Check sheet for the drawn part. Datum: minimum x, y, z corner. Units: mm. Round coordinates to 2 decimals unless told otherwise and drop trailing zeros. Write each loop counter-clockwise with the first axis right and the second up, starting at its lowest first coordinate (ties: lowest second). Pieces come first, ordered by that corner, then holes. Notation, with made-up numbers: (81.25, 68) - (87.25, 68) arc R8 ccw to (87.25, 79) - close; hole circle Ø9 at (37.25, -32). An arc over 180 degrees is marked (long way). Answer as a JSON object with one key per item and string values.
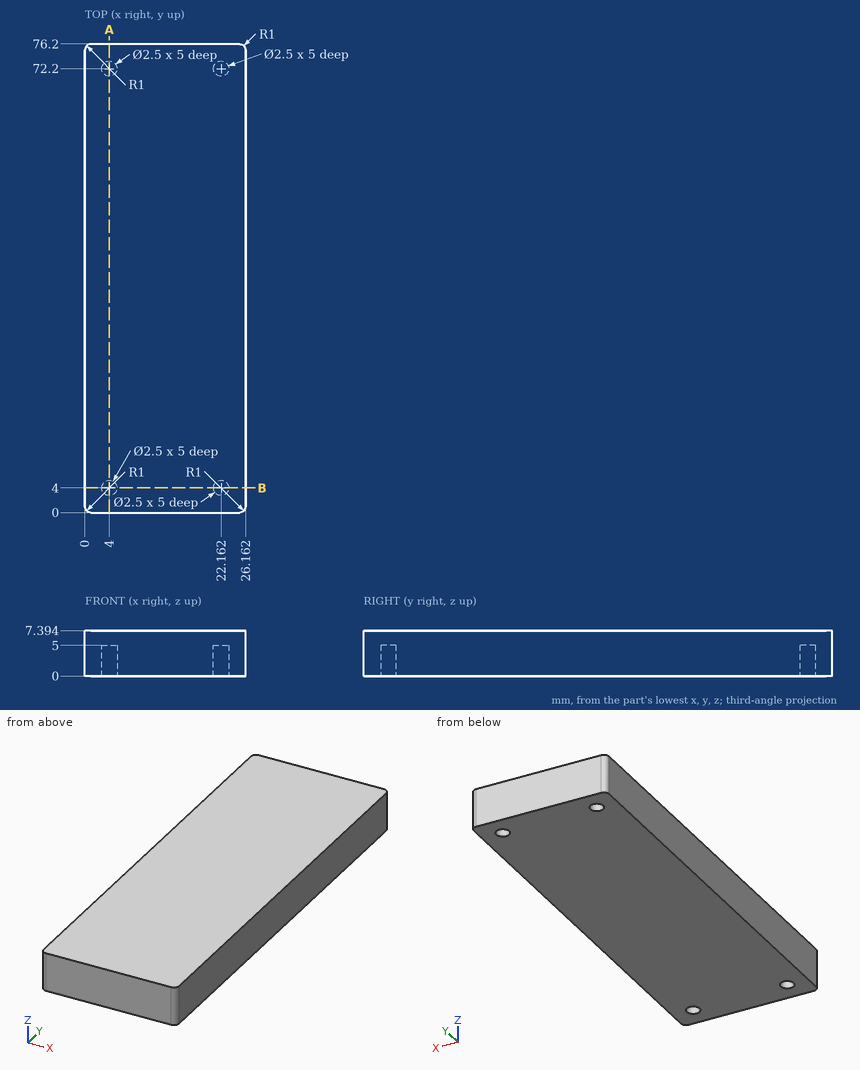
Q1. Section check A-A, the plane x = 4. Record the cut outline in (y, z).
Geometry check:
{"outline": "(0, 0) - (2.75, 0) - (2.75, 5) - (5.25, 5) - (5.25, 0) - (70.95, 0) - (70.95, 5) - (73.45, 5) - (73.45, 0) - (76.2, 0) - (76.2, 7.39) - (0, 7.39) - close"}
Q2. Gauge pin test, flat end, axial feed: P1, Ø2, axis at x = 4, y = 72.2, coming from the -Z side. Record the tip position at first contact, or that the pin passes through.
Geometry check:
{"P1": "stops at z = 5"}
Q3. Material ranges on line 1 along Y through (x, z) = (4, 2.8); line 2 along X through (y, z) = (72.2, 2.35), recorded low to high. Write a range as [from, to].
Geometry check:
{"line 1": "y = [0, 2.75], [5.25, 70.95], [73.45, 76.2]", "line 2": "x = [0, 2.75], [5.25, 20.91], [23.41, 26.16]"}
Q4. Section check B-B, the plane y = 4. Record the cut outline in (x, z).
Geometry check:
{"outline": "(0, 0) - (2.75, 0) - (2.75, 5) - (5.25, 5) - (5.25, 0) - (20.91, 0) - (20.91, 5) - (23.41, 5) - (23.41, 0) - (26.16, 0) - (26.16, 7.39) - (0, 7.39) - close"}
